from build123d import *

# Parameters (mm, degrees)
SKETCH_1_W               = 4.5
SKETCH_1_H               = 23
EXTRUDE_1_DEPTH          = 1.5
EXTRUDE_1_2_DEPTH        = 1.5
CUT_EXTRUDE_1_DEPTH      = 24.393375131
CUT_EXTRUDE_1_DEPTH_BACK = 24.393375131
SKETCH_2_R               = 1.65
SKETCH_4_W               = 3.5
SKETCH_4_H               = 3
EXTRUDE_3_DEPTH          = 23
SKETCH_5_W               = 32
SKETCH_5_H               = 3.5
EXTRUDE_4_DEPTH          = 31
SKETCH_6_W               = 32
SKETCH_6_H               = 3
EXTRUDE_5_DEPTH          = 20
SKETCH_8_R               = 3.35
EXTRUDE_6_DEPTH          = 6
CUT_EXTRUDE_2_REACH      = 36.205
SKETCH_9_R               = 1.5
SKETCH_10_W              = 18.606711353
SKETCH_10_H              = 21.185184653
CUT_EXTRUDE_3_DEPTH      = 44.179856415
SKETCH_11_W              = 7.069778579
SKETCH_11_H              = 20
CUT_EXTRUDE_4_DEPTH      = 10
FILLET_1_R               = 2


with BuildPart() as part:
    # Sketch 1 → Extrude 1 (new, symmetric)
    with BuildSketch(Plane(origin=(0, 0, 0), x_dir=(1, 0, 0), z_dir=(0, 1, 0))):
        with Locations((-13.75, 5.5)):
            Rectangle(SKETCH_1_W, SKETCH_1_H)
    extrude(amount=EXTRUDE_1_DEPTH, both=True)


with BuildPart() as body_2:
    # Sketch 1 → Extrude 1 2 (new, symmetric)
    with BuildSketch(Plane(origin=(0, 0, 0), x_dir=(1, 0, 0), z_dir=(0, 1, 0))):
        with Locations((13.75, 5.5)):
            Rectangle(SKETCH_1_W, SKETCH_1_H)
    extrude(amount=EXTRUDE_1_2_DEPTH, both=True)


with BuildPart() as cut_extrude_1_tool:
    # Sketch 2 → Cut-Extrude 1 (new, two sides: drawn at the far end of the back side and taken through both)
    with BuildSketch(Plane(origin=(0, 0, 0), x_dir=(1, 0, 0), z_dir=(0, 1, 0)).offset(-CUT_EXTRUDE_1_DEPTH_BACK)):
        with Locations(Location((-13.68, 0, 0), (0, 0, 270))):
            Circle(SKETCH_2_R)
        with Locations(Location((13.68, 0, 0), (0, 0, 270))):
            Circle(SKETCH_2_R)
    extrude(amount=CUT_EXTRUDE_1_DEPTH + CUT_EXTRUDE_1_DEPTH_BACK)


with BuildPart() as part_1:
    add(part.part)

    # Cut-Extrude 1: cut by cut_extrude_1_tool
    add(cut_extrude_1_tool.part, mode=Mode.SUBTRACT)



with BuildPart() as body_2_1:
    add(body_2.part)

    # Cut-Extrude 1: cut by cut_extrude_1_tool
    add(cut_extrude_1_tool.part, mode=Mode.SUBTRACT)


with BuildPart() as body_3:
    # Sketch 4 → Extrude 3 (new body)
    with BuildSketch(Plane(origin=(-11.5, 0, 0), x_dir=(0, 0, -1), z_dir=(1, 0, 0))):
        with Locations((15.25, 0)):
            Rectangle(SKETCH_4_W, SKETCH_4_H)
    extrude(amount=EXTRUDE_3_DEPTH)


with BuildPart() as part_2:
    add(part_1.part)

    add(body_2_1.part)  # Extrude 4 merges body 2

    add(body_3.part)  # Extrude 4 merges body 3
    # Sketch 5 → Extrude 4 (add)
    with BuildSketch(Plane(origin=(0, -1.5, 0), x_dir=(-1, 0, 0), z_dir=(0, -1, 0))):
        with Locations((0, 15.25)):
            Rectangle(SKETCH_5_W, SKETCH_5_H)
    extrude(amount=EXTRUDE_4_DEPTH)

    # Sketch 6 → Extrude 5 (add)
    with BuildSketch(Plane.XY.offset(-13.5)):
        with Locations((0, -31)):
            Rectangle(SKETCH_6_W, SKETCH_6_H)
    extrude(amount=EXTRUDE_5_DEPTH)

    # Sketch 8 → Extrude 6 (add)
    with BuildSketch(Plane(origin=(0, -29.5, 0), x_dir=(1, 0, 0), z_dir=(0, 1, 0))):
        with Locations(Location((5.15, 0, 0), (0, 0, 90))):
            Circle(SKETCH_8_R)
    extrude(amount=EXTRUDE_6_DEPTH)

    # Sketch 9 → Cut-Extrude 2 (cut, up to next)
    with BuildSketch(Plane(origin=(0, -23.5, 0), x_dir=(1, 0, 0), z_dir=(0, 1, 0)), mode=Mode.PRIVATE) as cut_extrude_2_sk1:
        with Locations(Location((5.15, 0, 0), (0, 0, 270))):
            Circle(SKETCH_9_R)
    cut_extrude_2_tool1 = extrude(cut_extrude_2_sk1.sketch, amount=-CUT_EXTRUDE_2_REACH, mode=Mode.PRIVATE) & part_2.part
    add(cut_extrude_2_tool1.solids().sort_by_distance((5.15, -23.5, 0))[0], mode=Mode.SUBTRACT)

    # Sketch 10 → Cut-Extrude 3 (cut, through all)
    with BuildSketch(Plane(origin=(0, 0, -17), x_dir=(-1, 0, 0), z_dir=(0, 0, -1))):
        with Locations((-0.324302099, -14.259789027)):
            Rectangle(SKETCH_10_W, SKETCH_10_H)
    extrude(amount=-CUT_EXTRUDE_3_DEPTH, mode=Mode.SUBTRACT)

    # Sketch 11 → Cut-Extrude 4 (cut)
    with BuildSketch(Plane(origin=(0, -29.5, 0), x_dir=(1, 0, 0), z_dir=(0, 1, 0))):
        with Locations((-12.46511071, 3.5)):
            Rectangle(SKETCH_11_W, SKETCH_11_H)
    extrude(amount=-CUT_EXTRUDE_4_DEPTH, mode=Mode.SUBTRACT)

    # Fillet 1
    fillet_1_edges = [part_2.edges().sort_by_distance(p)[0] for p in [
        (-13.75, -1.5, -13.5),
        (13.75, -1.5, -13.5),
        (3.534889289, -29.5, -13.5),
    ]]
    fillet(fillet_1_edges, radius=FILLET_1_R)


solid = part_2.part
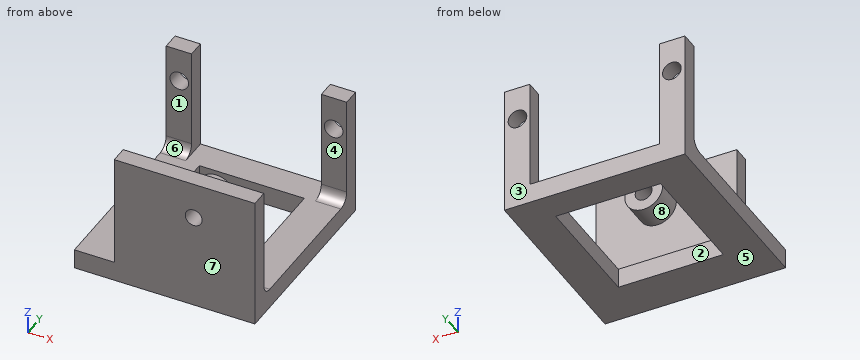
Read the model definition and answer for the solid it produces. Units are mm, in the model's axes. Face numbers are marked on the shaded views. A direction names the side the tool comes from. Round coordinates to 2 decimals unless told otherwise and drop trailing zeros. Order: outer loops, then holes, each group sorted by start corner. A loop starts at its lowest first (then second) coordinate and runs counter-clockwise, first axis right, second up. Notation, with made-up numbers: (-13.5, 12) - (41.5, 12) arc R33 ccw to (41.5, 47) - close; hole circle Ø3 at (81.25, 51.25). An arc over 180 degrees is marked (long way). Use one line per item in the form item = value. Start each with the question number.
(1) The part is cut by section D-D (z = -4.5). Give the vertices of the cut face in (x, y).
(2) The part is cut by section B-B (z = 0). Give the vertices of the cut face in (x, y), then the cut area to 3 significant figures.
(3) For the marked faces 1, 2, 3, 4 and 5, determine the directions among +Z, -Z, +X, -X, +Y, -Y from which every point of the face is accessible in a straight line to the end or side of a thin tool.
(4) Determine the mould class of the marked faces 6, 7 and 8 for opening direction Z: +Z half, -Z half, draft (parallel to the pull), parting line (faces both ways), or undercut.
(5) Flat-ended cylindrical pins translate along their axes: pin 1 Ø3.5 at (x, z) = (-13.5, -1.5) entering from -Y; pin 2 Ø9 at (x, z) = (5.5, -5.5) entering from +Y; pin 3 Ø10 at (x, y) = (-0.5, -13) entering from +Z; pin 4 Ø0.9 at (x, y) = (13, 0.5) entering from +Z. Find the tip coordinate at first contact, or state that the pin passes through.
(6) Find the intervals of material crossed by line 1 along X through (y, z) = (-0.15, 0); line 2 along Z through (x, y) = (13.68, -0.1); line 3 along Z through (x, y) = (13, 0), in increasing order. Write a range as from..to.
(7) The part is cut by section A-A (x = -13.68). Give the vertices of the cut face in (y, z).
(8) The part is cut by section C-C (y = -13). Give the vertices of the cut face in (x, z), then the cut area to 3 significant figures.
Checked values:
q1.outline = (-16, -1.5) - (-11.5, -1.5) - (-11.5, 1.5) - (-16, 1.5) - close; (-8.93, -32.5) - (16, -32.5) - (16, -29.5) - (-8.93, -29.5) - close; (11.5, -1.5) - (16, -1.5) - (16, 1.5) - (11.5, 1.5) - close
q2.outline = (-16, -1.5) - (-15.33, -1.5) - (-15.33, 1.5) - (-16, 1.5) - close; (-12.03, -1.5) - (-11.5, -1.5) - (-11.5, 1.5) - (-12.03, 1.5) - close; (-8.93, -32.5) - (3.65, -32.5) - (3.65, -24.85) - (1.8, -24.85) - (1.8, -29.5) - (-8.93, -29.5) - close; (6.65, -32.5) - (16, -32.5) - (16, -29.5) - (8.5, -29.5) - (8.5, -24.85) - (6.65, -24.85) - close; (11.5, -1.5) - (12.03, -1.5) - (12.03, 1.5) - (11.5, 1.5) - close; (15.33, -1.5) - (16, -1.5) - (16, 1.5) - (15.33, 1.5) - close
q2.area = 90.2 mm^2
q3.face_1 = +Z, +X, -X, -Y
q3.face_2 = +Z, -Z
q3.face_3 = +Z, -Z, +X, -X, +Y
q3.face_4 = +Z, +X, -X
q3.face_5 = -Z, +X, -X, +Y, -Y
q4.face_6 = +Z half
q4.face_7 = draft
q4.face_8 = undercut
q5.pin_1 = -1.5
q5.pin_2 = -24.85
q5.pin_3 = through
q5.pin_4 = 6
q6.line_1 = -16..-15.33, -12.03..-11.5, 11.5..12.03, 15.33..16
q6.line_2 = -17..-1.65, 1.65..6
q6.line_3 = -17..-1.5, 1.5..6
q7.outline = (-32.5, -17) - (1.5, -17) - (1.5, -1.65) - (-1.5, -1.65) - (-1.5, -11.5) arc R2 cw to (-3.5, -13.5) - (-32.5, -13.5) - close; (-1.5, 1.65) - (1.5, 1.65) - (1.5, 6) - (-1.5, 6) - close
q8.outline = (-16, -17) - (-8.98, -17) - (-8.98, -13.5) - (-16, -13.5) - close; (9.63, -17) - (16, -17) - (16, -13.5) - (9.63, -13.5) - close
q8.area = 46.9 mm^2
